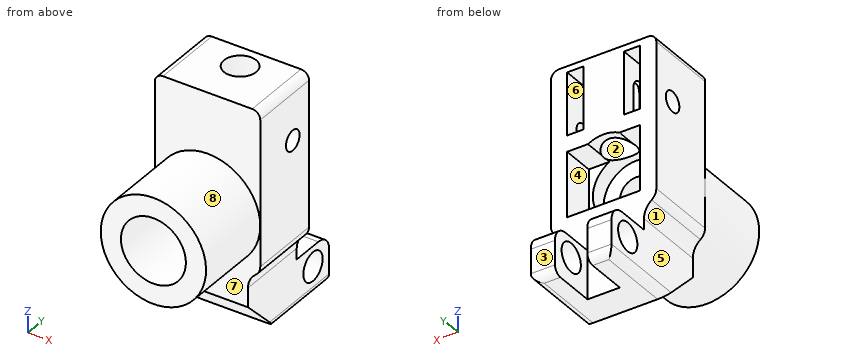
```python
from build123d import *

# Parameters (mm, degrees)
SKETCH1_R               = 13.05
SKETCH1_R_2             = 8.05
BOSS_EXTRUDE1_DEPTH     = 20
SKETCH2_R               = 8.05
BOSS_EXTRUDE2_DEPTH     = 10
SKETCH3_W               = 18.1
SKETCH3_H               = 13
CUT_EXTRUDE1_DEPTH      = 4
SKETCH4_W               = 18.1
SKETCH4_H               = 13
BOSS_EXTRUDE3_DEPTH     = 8
SKETCH5_R               = 8.05
SKETCH5_R_2             = 4
BOSS_EXTRUDE4_DEPTH     = 6
SKETCH10_W              = 10.1
SKETCH10_H              = 13
BOSS_EXTRUDE7_DEPTH     = 12
CUT_EXTRUDE2_REACH      = 59.476
SKETCH6_R               = 4
CUT_EXTRUDE3_DEPTH      = 54.963066195
CUT_EXTRUDE3_DEPTH_BACK = 54.963066195
SKETCH7_R               = 2.5
BOSS_EXTRUDE5_DEPTH     = 10
SKETCH13_W              = 6
SKETCH13_H              = 12
BOSS_EXTRUDE8_DEPTH     = 12
FILLET1_R               = 5
FILLET2_R               = 2
CUT_EXTRUDE4_REACH      = 63.577
CUT_EXTRUDE5_REACH      = 65.209
SKETCH14_R              = 3.55
FILLET4_R               = 4
FILLET5_R               = 2
SKETCH15_W              = 4
SKETCH15_H              = 2.5
CUT_EXTRUDE6_DEPTH      = 12


with BuildPart() as part:
    # Sketch1 → Boss-Extrude1 (new body)
    with BuildSketch(Plane(origin=(0, 0, 0), x_dir=(1, 0, 0), z_dir=(0, 1, 0))):
        with Locations(Location((0, 0, 0), (0, 0, 270))):
            Circle(SKETCH1_R)
        with Locations(Location((0, 0, 0), (0, 0, 270))):
            Circle(SKETCH1_R_2, mode=Mode.SUBTRACT)
    extrude(amount=BOSS_EXTRUDE1_DEPTH)

    # Sketch2 → Boss-Extrude2 (add)
    with BuildSketch(Plane(origin=(0, 20, 0), x_dir=(1, 0, 0), z_dir=(0, 1, 0))):
        with BuildLine():
            Line((-13.05, -13.05), (-13.05, 10))
            ThreePointArc((-13.05, 10), (-12.156675683, 12.156675683), (-10, 13.05))
            Line((-10, 13.05), (10, 13.05))
            ThreePointArc((10, 13.05), (12.156675683, 12.156675683), (13.05, 10))
            Line((13.05, 10), (13.05, -13.05))
            Line((13.05, -13.05), (13.05, -28.05))
            Line((13.05, -28.05), (-13.05, -28.05))
            Line((-13.05, -28.05), (-13.05, -13.05))
        make_face()
        with Locations(Location((0, 0, 0), (0, 0, 270))):
            Circle(SKETCH2_R, mode=Mode.SUBTRACT)
    extrude(amount=BOSS_EXTRUDE2_DEPTH)

    # Sketch3 → Cut-Extrude1 (cut)
    with BuildSketch(Plane(origin=(0, 30, 0), x_dir=(1, 0, 0), z_dir=(0, 1, 0))):
        with Locations((0, -17.55)):
            Rectangle(SKETCH3_W, SKETCH3_H)
    extrude(amount=-CUT_EXTRUDE1_DEPTH, mode=Mode.SUBTRACT)

    # Sketch4 → Boss-Extrude3 (add)
    with BuildSketch(Plane(origin=(0, 30, 0), x_dir=(1, 0, 0), z_dir=(0, 1, 0))):
        with BuildLine():
            Line((-13.05, -28.05), (13.05, -28.05))
            Line((13.05, -28.05), (13.05, 10))
            ThreePointArc((13.05, 10), (12.156675683, 12.156675683), (10, 13.05))
            Line((10, 13.05), (-10, 13.05))
            ThreePointArc((-10, 13.05), (-12.156675683, 12.156675683), (-13.05, 10))
            Line((-13.05, 10), (-13.05, -28.05))
        make_face()
        with BuildLine():
            Line((-9.05, 9.05), (-9.05, -7.05))
            Line((-9.05, -7.05), (-3.885871846, -7.05))
            ThreePointArc((-3.885871846, -7.05), (0, -8.05), (3.885871846, -7.05))
            Line((3.885871846, -7.05), (9.05, -7.05))
            Line((9.05, -7.05), (9.05, 9.05))
            Line((9.05, 9.05), (-9.05, 9.05))
        make_face(mode=Mode.SUBTRACT)
        with Locations((0, -17.55)):
            Rectangle(SKETCH4_W, SKETCH4_H, mode=Mode.SUBTRACT)
    extrude(amount=BOSS_EXTRUDE3_DEPTH)

    # Sketch5 → Boss-Extrude4 (add)
    with BuildSketch(Plane(origin=(0, 20, 0), x_dir=(1, 0, 0), z_dir=(0, 1, 0))):
        with Locations(Location((0, 0, 0), (0, 0, 270))):
            Circle(SKETCH5_R)
        with Locations(Location((0, 0, 0), (0, 0, 270))):
            Circle(SKETCH5_R_2, mode=Mode.SUBTRACT)
    extrude(amount=BOSS_EXTRUDE4_DEPTH)

    # Sketch10 → Boss-Extrude7 (add)
    with BuildSketch(Plane(origin=(0, 26, 0), x_dir=(1, 0, 0), z_dir=(0, 1, 0))):
        with Locations((0, -17.55)):
            Rectangle(SKETCH10_W, SKETCH10_H)
    extrude(amount=BOSS_EXTRUDE7_DEPTH)

    # Cut-Extrude2: up to this face of the body (flat: up to its plane)
    cut_extrude2_end = Plane(part.part.faces().sort_by_distance((-6.467935923, 34, 7.05))[0])
    # Sketch6 → Cut-Extrude2 (cut, up to the picked face)
    with BuildSketch(Plane.XY.offset(28.05), mode=Mode.PRIVATE) as cut_extrude2_sk1:
        with Locations((0, 32)):
            Circle(SKETCH6_R)
    cut_extrude2_tool1 = split(extrude(cut_extrude2_sk1.sketch, amount=-CUT_EXTRUDE2_REACH, mode=Mode.PRIVATE), bisect_by=cut_extrude2_end, keep=Keep.BOTH, mode=Mode.PRIVATE)
    add(cut_extrude2_tool1.solids().sort_by(Axis((0, 32, 28.05), (0, 0, -1)))[0], mode=Mode.SUBTRACT)

    # Sketch7 → Cut-Extrude3 (cut, two sides: drawn at the far end of the back side and taken through both)
    with BuildSketch(Plane(origin=(13.05, 0, 0), x_dir=(0, 0, -1), z_dir=(1, 0, 0)).offset(-CUT_EXTRUDE3_DEPTH_BACK)):
        with Locations((-14.55, 32)):
            Circle(SKETCH7_R)
    extrude(amount=CUT_EXTRUDE3_DEPTH + CUT_EXTRUDE3_DEPTH_BACK, mode=Mode.SUBTRACT)

    # Sketch8 → Boss-Extrude5 (add, symmetric)
    with BuildSketch(Plane(origin=(0, 0, 0), x_dir=(0, 0, -1), z_dir=(1, 0, 0))):
        Polygon((21.05, 20), (31.05, 30), (31.05, 38), (13.05, 38), (13.05, 20), align=None)
    extrude(amount=BOSS_EXTRUDE5_DEPTH, both=True)

    # Sketch13 → Boss-Extrude8 (add)
    with BuildSketch(Plane(origin=(0, 38, 0), x_dir=(1, 0, 0), z_dir=(0, 1, 0))):
        with Locations((-7, 25.05)):
            Rectangle(SKETCH13_W, SKETCH13_H)
        with Locations((7, 25.05)):
            Rectangle(SKETCH13_W, SKETCH13_H)
    extrude(amount=BOSS_EXTRUDE8_DEPTH)

    # Fillet1
    fillet1_edges = [part.edges().sort_by_distance(p)[0] for p in [
        (10, 29, -13.05),
        (-10, 29, -13.05),
    ]]
    fillet(fillet1_edges, radius=FILLET1_R)

    # Fillet2
    fillet2_edges = [part.edges().sort_by_distance(p)[0] for p in [
        (-10, 40, -31.05),
        (10, 40, -31.05),
        (-7, 50, -31.05),
        (7, 50, -31.05),
    ]]
    fillet(fillet2_edges, radius=FILLET2_R)

    # Cut-Extrude4: up to this face of the body (flat: up to its plane)
    cut_extrude4_end = Plane(part.part.faces().sort_by_distance((-5.05, 32, 17.981964525))[0])
    # Sketch11 → Cut-Extrude4 (cut, up to the picked face)
    with BuildSketch(Plane(origin=(5.05, 0, 0), x_dir=(0, 0, -1), z_dir=(1, 0, 0)), mode=Mode.PRIVATE) as cut_extrude4_sk1:
        with BuildLine():
            Line((-19.75, 29.5), (-14.55, 29.5))
            ThreePointArc((-14.55, 29.5), (-12.05, 32), (-14.55, 34.5))
            Line((-14.55, 34.5), (-19.75, 34.5))
            ThreePointArc((-19.75, 34.5), (-22.25, 32), (-19.75, 29.5))
        make_face()
    cut_extrude4_tool1 = split(extrude(cut_extrude4_sk1.sketch, amount=-CUT_EXTRUDE4_REACH, mode=Mode.PRIVATE), bisect_by=cut_extrude4_end, keep=Keep.BOTH, mode=Mode.PRIVATE)
    add(cut_extrude4_tool1.solids().sort_by(Axis((5.05, 32, 17.15), (-1, 0, 0)))[0], mode=Mode.SUBTRACT)

    # Cut-Extrude5: up to this face of the body (flat: up to its plane)
    cut_extrude5_end = Plane(part.part.faces().sort_by_distance((-10, 35.310803733, -22.824229644))[0])
    # Sketch14 → Cut-Extrude5 (cut, up to the picked face)
    with BuildSketch(Plane(origin=(10, 0, 0), x_dir=(0, 0, -1), z_dir=(1, 0, 0)), mode=Mode.PRIVATE) as cut_extrude5_sk1:
        with Locations((24.05, 44)):
            Circle(SKETCH14_R)
    cut_extrude5_tool1 = split(extrude(cut_extrude5_sk1.sketch, amount=-CUT_EXTRUDE5_REACH, mode=Mode.PRIVATE), bisect_by=cut_extrude5_end, keep=Keep.BOTH, mode=Mode.PRIVATE)
    add(cut_extrude5_tool1.solids().sort_by(Axis((10, 44, -24.05), (-1, 0, 0)))[0], mode=Mode.SUBTRACT)

    # Fillet4
    fillet4_edges = [part.edges().sort_by_distance(p)[0] for p in [
        (-7, 50, -19.05),
        (7, 50, -19.05),
    ]]
    fillet(fillet4_edges, radius=FILLET4_R)

    # Fillet5
    fillet5_edges = [part.edges().sort_by_distance(p)[0] for p in [
        (-13.05, 29, 28.05),
        (13.05, 29, 28.05),
    ]]
    fillet(fillet5_edges, radius=FILLET5_R)

    # Sketch15 → Cut-Extrude6 (cut)
    with BuildSketch(Plane(origin=(0, 38, 0), x_dir=(1, 0, 0), z_dir=(0, 1, 0))):
        with Locations((7.05, -25.3)):
            Rectangle(SKETCH15_W, SKETCH15_H)
        with Locations((-7.05, -25.3)):
            Rectangle(SKETCH15_W, SKETCH15_H)
    extrude(amount=-CUT_EXTRUDE6_DEPTH, mode=Mode.SUBTRACT)


solid = part.part
```
Here's how the part is built. I have some questions about the finished solid (model axes, mm). Face numbers are marked on the shaded views. A direction names the side the tool comes from. Round coordinates to 2 decimals unless told otherwise and drop trailing zeros. Loops run counter-clockwise (first coordinate to the right, second up) from the corner with the lowest first, then second, coordinate; pieces in that order, holes last. Notation, with made-up numbers: (28, 13) -> (32, 13) arc R4 cw to (32, 19) -> close; hole circle Ø3 at (7, 61.5). An arc over 180 degrees is marked (long way). Answer as CSV lines item,"result". Start each with the question number.
1. For the marked faces 5, 6, 7 and 8, which set-ups out of +Z, -Z, +X, -X, +Y, -Y let a thin tool reach every point of the face, with its end or its side?
2. Imagine slicing it at D-D on y = 32. State how many separate pieces and enclosed holes the cut face has, plus the area to 3 significant figures.
3. I need wall thicknesses on probe 1 along Y at (x, z) = (0, 12.5); probe 2 along X at (y, z) = (7, 0); probe 3 along X at (y, z) = (33, -6). Which ranges of each line are inside material? Lowest first, please. Write a range as from..to.
4. I'm going to push flat-ended pins straight in: P1, Ø8, axis at x = -0.5, z = -2, coming from the +Y side; P2, Ø10, axis at y = 34.5, z = -24, coming from the -X side; P3, Ø2.5, axis at x = 0, y = 34.5, coming from the +Z side. Where does each tip first touch, or does it pass through?
5. Imagine slicing it at B-B on y = 24. Write out the boundary of the cut face in (x, z), plus the area to 3 significant figures.
6. Imagine slicing it at A-A on x = 0. Write out the boundary of the cut face in (y, z).
7. If we mould it in two halves opening along X, with no side actions, what happens to the marked faces 1, 2, 3 and 4? For each: pulls with the +X half, pulls with the -X half, needs draft (parallel to the pull), parting line crosses it, or undercut.
Solution:
1,face 5,"-Z, -X, +Y, -Y"
1,face 6,"+Y"
1,face 7,"-Z, -Y"
1,face 8,"-Y"
2,separate pieces,"3"
2,enclosed holes,"0"
2,area,"783 mm²"
3,probe 1,"0..28, 36..38"
3,probe 2,"-13.05..-8.05, 8.05..13.05"
3,probe 3,"-13.05..-9.05, 9.05..13.05"
4,P1,"y = 26"
4,P2,"x = -10"
4,P3,"z = -9.05"
5,outline,"(-13.05, -10) arc R3.05 ccw to (-11.89, -12.39) arc R5 cw to (-10, -16.31) -> (-10, -25.05) -> (10, -25.05) -> (10, -16.31) arc R5 cw to (11.89, -12.39) arc R3.05 ccw to (13.05, -10) -> (13.05, 26.05) arc R2 ccw to (11.05, 28.05) -> (-11.05, 28.05) arc R2 ccw to (-13.05, 26.05) -> close; hole circle Ø8 at (0, 0)"
5,area,"1,260 mm²"
6,outline,"(0, -13.05) -> (20, -13.05) -> (20, -21.05) -> (30, -31.05) -> (38, -31.05) -> (38, -9.05) -> (30, -9.05) -> (30, -8.05) -> (26, -8.05) -> (26, -4) -> (20, -4) -> (20, -8.05) -> (0, -8.05) -> close; (0, 8.05) -> (20, 8.05) -> (20, 4) -> (26, 4) -> (26, 8.05) -> (28, 8.05) -> (28, 28.05) -> (20, 28.05) -> (20, 13.05) -> (0, 13.05) -> close; (36, 8.05) -> (38, 8.05) -> (38, 28.05) -> (36, 28.05) -> close"
7,face 1,"pulls with the -X half"
7,face 2,"undercut"
7,face 3,"needs draft"
7,face 4,"undercut"
